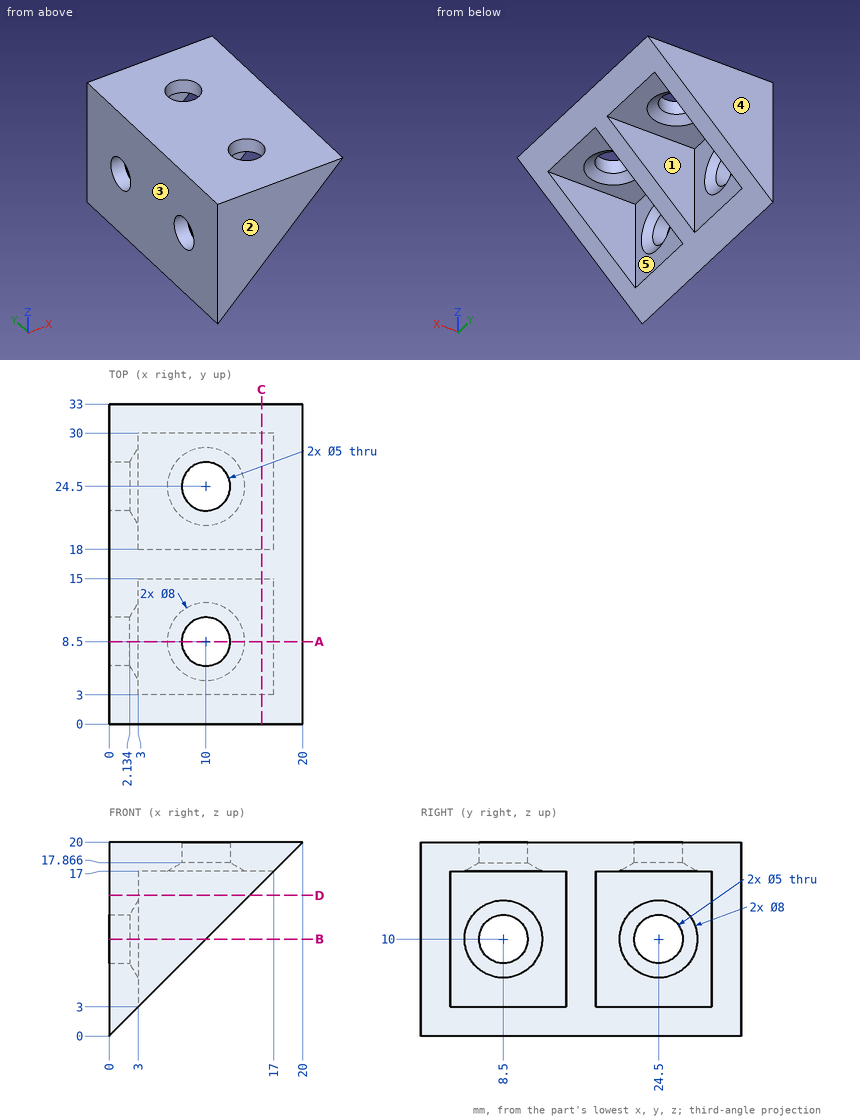
Source: three-view drawing plus pictorial views. Frame: mm from the lowest corner of the part. A direction names the side the tool comes from. Round coordinates to 2 decimals unless told otherwise and drop trailing zeros. Write each loop counter-clockwise with the first axis right and the second up, starting at its lowest first coordinate (ties: lowest second). Pieces come first, ordered by that corner, then holes. Notation, with made-up numbers: M 70,19.5 L 88,19.5 A28 cw 88,41.5 Z; hole C 45.25,-17 d5. An arc over 180 degrees is marked long. Write item = value, one per line.
Item 1: Pin query (flat end, axial travel): P1, Ø3, axis at x = 10, y = 24.5, coming from the +Z side; P2, Ø6.5, axis at y = 24.5, z = 10, coming from the +X side; P3, Ø9.5, axis at x = 12.5, y = 23, coming from the -Z side; P4, Ø2, axis at y = 6.5, z = 4, coming from the +X side. Return the tip coordinate at first contact, or that it passes through.
Findings:
P1 = through
P2 = 2.57
P3 = 17
P4 = 3
Item 2: Section query B-B on z = 10. Return loops of the section in (x, y), then the cut area to 3 significant figures.
Findings:
outline = M 0,0 L 10,0 L 10,3 L 3,3 L 3,4.5 L 2.13,6 L 0,6 Z; M 0,11 L 2.13,11 L 3,12.5 L 3,15 L 10,15 L 10,18 L 3,18 L 3,20.5 L 2.13,22 L 0,22 Z; M 0,27 L 2.13,27 L 3,28.5 L 3,30 L 10,30 L 10,33 L 0,33 Z
area = 129 mm^2
Item 3: Material intervals for line 1 along Y through (x, z) = (0.65, 10); line 2 along Y through (x, z) = (4.5, 12.5); line 3 along Z through (x, y) = (1.2, 8.5), sorted ascending. Write a range as [from, to].
Findings:
line_1 = [0, 6], [11, 22], [27, 33]
line_2 = [0, 3], [15, 18], [30, 33]
line_3 = [1.2, 7.5], [12.5, 20]
Item 4: Section query D-D on z = 14.5. Return loops of the section in (x, y).
Findings:
outline = M 0,0 L 14.5,0 L 14.5,3 L 3,3 L 3,15 L 14.5,15 L 14.5,18 L 3,18 L 3,30 L 14.5,30 L 14.5,33 L 0,33 Z
Item 5: Pull-direction query (Y, two-part tool) for the marked faces 1, 2 and 3; classes: pulls with the +Y half, pulls with the -Y half, needs draft (parallel to the pull), parting line crosses it, or undercut.
Findings:
face_1 = undercut
face_2 = pulls with the -Y half
face_3 = needs draft
Item 6: Access query for the marked faces 4 and 5. Directions: +Z, -Z, +X, -X, +Y, -Y. A direction counts if a zero-diameter tool reaches every point of the face in a straight line with its end or side. Return the directions, or none.
Findings:
face_4 = +Z, -Z, +X, -X, +Y
face_5 = -Z, +X
Item 7: Section query C-C on x = 15.75. Return loops of the section in (y, z).
Findings:
outline = M 0,15.75 L 3,15.75 L 3,17 L 15,17 L 15,15.75 L 18,15.75 L 18,17 L 30,17 L 30,15.75 L 33,15.75 L 33,20 L 0,20 Z
Item 8: Section query A-A on y = 8.5. Return loops of the section in (x, z).
Findings:
outline = M 0,0 L 3,3 L 3,6 L 2.13,7.5 L 0,7.5 Z; M 0,12.5 L 2.13,12.5 L 3,14 L 3,17 L 6,17 L 7.5,17.87 L 7.5,20 L 0,20 Z; M 12.5,17.87 L 14,17 L 17,17 L 20,20 L 12.5,20 Z
